Model file for the job. Use its own axes, mm. Face numbers are marked on the shaded views. Give positions to 0.01 mm unless a question says otherwise; leave off trailing zeros. Loops run counter-clockwise (first coordinate to the right, second up) from the corner with the lowest first, then second, coordinate; pieces in that order, holes last. Notation, with made-up numbers: (-28, 46) -> (-6, 46) arc R23 ccw to (-6, 70) -> close; hole circle Ø1 at (89.5, 25.5). An arc over 180 degrees is marked (long way). Use CSV: the item, a comma, the result in double quotes. Start each with the question number.
(1) Drill centre lines: probe 1 along Z at (x, y) = (-3, 8.25); probe 2 along Y at (x, z) = (-5.5, 86). Where is each one in solid material? Low to high.
(2) Flat gauge pins, fed straight in: pin 1 (6 mm diameter, centred on x = -7, y = -5.5, fed in from -Z); pin 2 (10 mm diameter, centred on x = -0.5, z = 104, fed in from +Y). Where does each tip first touch, or does it go through?
(3) Cut at B-B on z = 105. Write the cut outline in (x, y), then the cut area to 3 significant figures.
(4) Cut at A-A on x = 4.75. Write the cut outline in (y, z).
(5) Pull direction Z, two halves, no side cores. Call the marked faces 1 and 2: pulls with the +Z half, pulls with the -Z half, needs draft (parallel to the pull), parting line crosses it, or undercut.
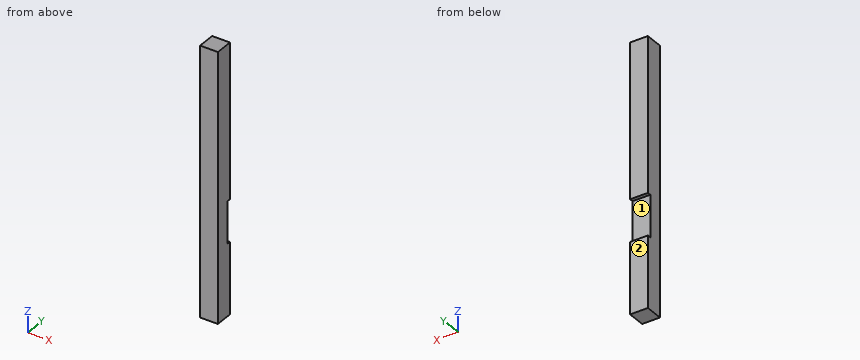
Autodesk Inventor part; units mm, degrees
ref_plane "YZ Plane" through (0, 0, 0) normal (1, 0, 0) x (0, 1, 0)
ref_plane "XZ Plane" through (0, 0, 0) normal (0, 1, 0) x (-1, 0, 0)
ref_plane "XY Plane" through (0, 0, 0) normal (0, 0, 1) x (1, 0, 0)
sketch "Sketch1" plane through (0, 0, 0) normal (0, 0, 1) x (1, 0, 0)
  line L0 (-10, 10) -> (10, 10)
  line L1 (10, 10) -> (10, -10)
  line L2 (10, -10) -> (-10, -10)
  line L3 (-10, -10) -> (-10, 10)
  point P0 (0, 0)
  dimension "d0" = 20
  dimension "d1" = 20
  dimension "d2" = 10
  dimension "d3" = 10
extrude "Extrusion1" add sketch "Sketch1" along normal blind 300
sketch "Sketch2" plane through (-10, 10, 0) normal (0, 1, 0) x (1, 0, 0)
  line L0 (0, 0) -> (0, -300)
  line L1 (20, 0) -> (20, -300)
  line L2 (0, -127) -> (20, -127)
  line L3 (20, -127) -> (20, -80)
  line L4 (20, -80) -> (0, -80)
  line L5 (0, -80) -> (0, -127)
  line L6 (0, 0) -> (20, 0)
  point P0 (10, 0)
  dimension "d6" = 47
  dimension "d7" = 80
extrude "Extrusion2" cut sketch "Sketch2" against normal blind 4 contours L4 L1 L2 L0
properties part number "cnc power plug"
Check result:
1,probe 1,"0 to 80, 127 to 300"
1,probe 2,"-10 to 6"
2,pin 1,"z = 0"
2,pin 2,"y = 6"
3,outline,"(-10, -10) -> (10, -10) -> (10, 6) -> (-10, 6) -> close"
3,area,"320 mm²"
4,outline,"(-10, 0) -> (10, 0) -> (10, 80) -> (6, 80) -> (6, 127) -> (10, 127) -> (10, 300) -> (-10, 300) -> close"
5,face 1,"undercut"
5,face 2,"needs draft"
